The figure shows three views and two pictorial views of one solid part (mm, origin at its lowest corner). Answer the questions. Give positions to 0.01 mm unless a question says otherwise; leave off trailing zeros. Order: outer loops, then holes, each group sorted by start corner. A loop starts at its lowest first (then second) coordinate and runs counter-clockwise, first axis right, second up. Notation, with made-up numbers: M 33.25,-5.75 L 65.25,-5.75 A28 ccw 65.25,18.25 Z; hole C 30,73.25 d3. An arc over 180 degrees is marked long. Write item = value, one per line. Start each with the question number.
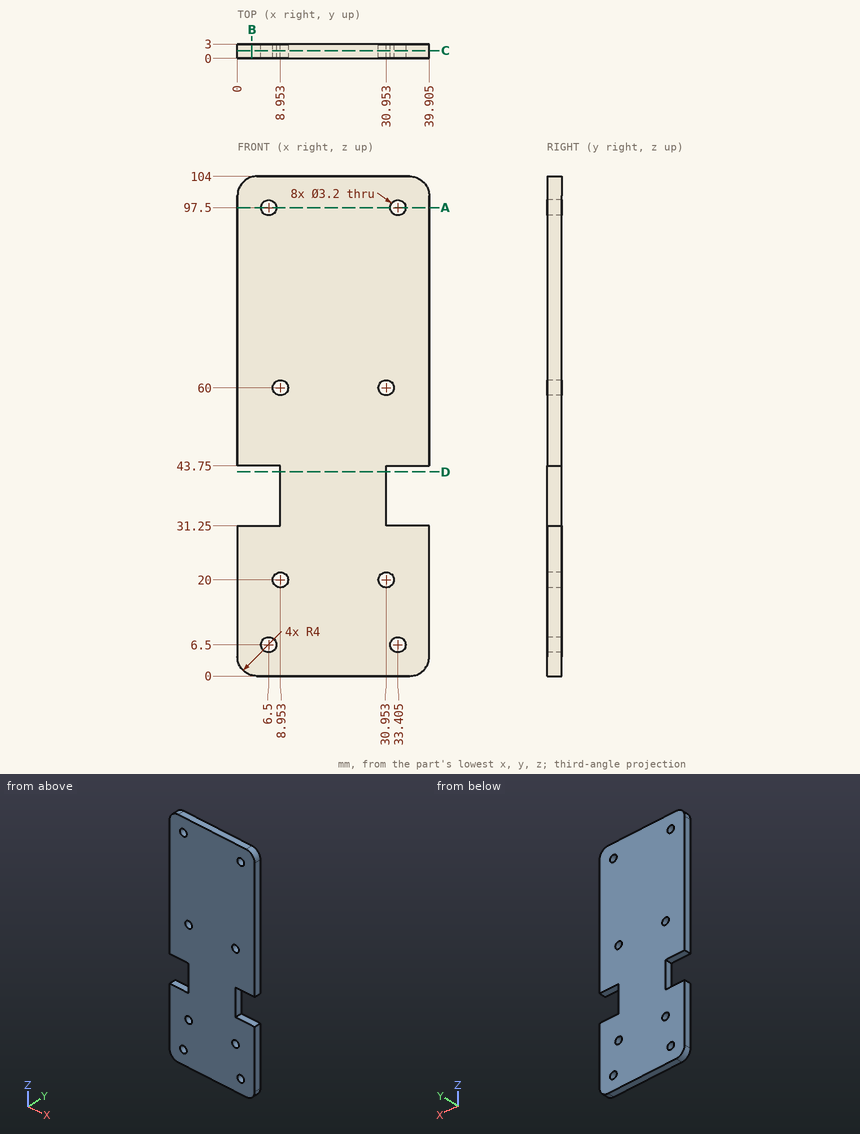
1) Each of these flat-tipped pins is pushed along its axis until it touches: P1, Ø1.5, axis at y = 1.5, z = 37, coming from the -X side; P2, Ø0.9, axis at x = 2.5, y = 2, coming from the -Z side. Where does it stop, or does it pass through?
2) Find the intervals of material crossed by probe 1 along X at (y, z) = (1.6, 97.5) (1 decimal); probe 2 along Z at (x, y) = (6.5, 2.35); probe 3 along Z at (x, y) = (3, 2.65), in increasing order. Write a range as [from, to].
3) Find section A-A on z = 97.5. Determine the outline of the cut face in (x, y) (1 decimal).
4) Find section C-C on y = 1.6. Count the separate pieces of the cut face and the enclosed holes in it, plus the area to 3 significant figures.
5) Find section B-B on x = 3. Determine the outline of the cut face in (y, z), plus the area to 3 significant figures.
6) Find section D-D on z = 42.5. Determine the outline of the cut face in (x, y).
Numbers:
q1.P1 = 8.95
q1.P2 = 0.14
q2.probe_1 = [0, 4.9], [8.1, 31.8], [35, 39.9]
q2.probe_2 = [0, 4.9], [8.1, 31.25], [43.75, 95.9], [99.1, 104]
q2.probe_3 = [0.13, 31.25], [43.75, 103.87]
q3.outline = M 0,0 L 4.9,0 L 4.9,3 L 0,3 Z; M 8.1,0 L 31.8,0 L 31.8,3 L 8.1,3 Z; M 35,0 L 39.9,0 L 39.9,3 L 35,3 Z
q4.separate_pieces = 1
q4.enclosed_holes = 8
q4.area = 3,850 mm2
q5.outline = M 0,0.13 L 3,0.13 L 3,31.25 L 0,31.25 Z; M 0,43.75 L 3,43.75 L 3,103.87 L 0,103.87 Z
q5.area = 274 mm2
q6.outline = M 8.95,0 L 30.95,0 L 30.95,3 L 8.95,3 Z
